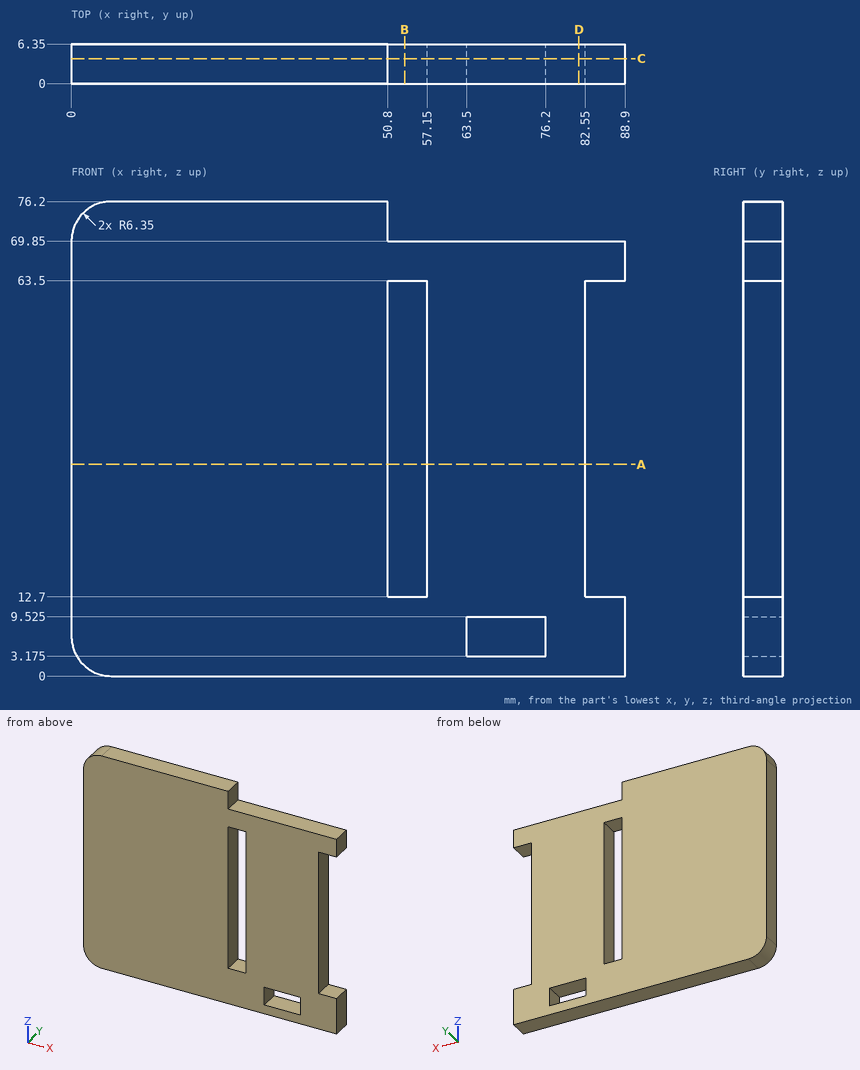
Geometry check sheet. Reference: drawing and pictorial views, mm from the part's lowest x, y, z. Give positions to 0.01 mm unless a question says otherwise; leave off trailing zeros. Write each loop counter-clockwise with the first axis right and the second up, starting at its lowest first coordinate (ties: lowest second). Pieces come first, ordered by that corner, then holes. Notation, with made-up numbers: M 84.5,-22.5 L 127.5,-22.5 A19 ccw 127.5,-17.5 Z; hole C 16,44.25 d4. An arc over 180 degrees is marked long. Answer as CSV lines item,"result". Start each with the question number.
Q1. Section check C-C, the plane y = 4. Record the cut outline in (x, z) (3 decimals).
Q2. Go/stop test with flat-tipped pins: pin 1 (1.5 mm diameter, centred on y = 2.5, z = 66.5, fed in from -X); pin 2 (3 mm diameter, centred on y = 4.5, z = 40.5, fed in from +X); pin 3 (1.9 mm diameter, centred on x = 71.5, y = 3, fed in from +Z); pin 4 (1.9 mm diameter, centred on y = 4.5, z = 74.5, fed in from +X). Record where each tip stops, or that it passes through.
Q3. Section check D-D, the plane x = 81.5. Record the cut outline in (y, z).
Q4. Section check B-B, the plane x = 53.5. Record the cut outline in (y, z), then the cut area to 3 significant figures.
Q5. Material ranges on L1, parallel to X at y = 1.25, z = 47; L2, parallel to Z at x = 72, y = 4.75 (3 decimals); L3, parallel to Z at x = 52.5, y = 3.5, recorded low to high.
Q6. Section check A-A, the plane z = 34. Record the cut outline in (x, y), then the cut area to 3 significant figures.
Geometry says:
1,outline,"M 0,6.35 A6.35 ccw 6.35,0 L 88.9,0 L 88.9,12.7 L 82.55,12.7 L 82.55,63.5 L 88.9,63.5 L 88.9,69.85 L 50.8,69.85 L 50.8,76.2 L 6.35,76.2 A6.35 ccw 0,69.85 Z; hole M 50.8,12.7 L 57.15,12.7 L 57.15,63.5 L 50.8,63.5 Z; hole M 63.5,3.175 L 76.2,3.175 L 76.2,9.525 L 63.5,9.525 Z"
2,pin 1,"x = 0"
2,pin 2,"x = 82.55"
2,pin 3,"z = 69.85"
2,pin 4,"x = 50.8"
3,outline,"M 0,0 L 6.35,0 L 6.35,69.85 L 0,69.85 Z"
4,outline,"M 0,0 L 6.35,0 L 6.35,12.7 L 0,12.7 Z; M 0,63.5 L 6.35,63.5 L 6.35,69.85 L 0,69.85 Z"
4,area,"121 mm^2"
5,L1,"0 to 50.8, 57.15 to 82.55"
5,L2,"0 to 3.175, 9.525 to 69.85"
5,L3,"0 to 12.7, 63.5 to 69.85"
6,outline,"M 0,0 L 50.8,0 L 50.8,6.35 L 0,6.35 Z; M 57.15,0 L 82.55,0 L 82.55,6.35 L 57.15,6.35 Z"
6,area,"484 mm^2"
